```python
from build123d import *

# Parameters (mm, degrees)
F0_R     = 11
F0_R_2   = 5.5
F0_R_3   = 4
F0_R_4   = 2.9
F1_DEPTH = 1.5
F2_DEPTH = 1.65
F3_DEPTH = 5


with BuildPart() as f1:
    # F0 (on Front) → F1 (new body)
    with BuildSketch(Plane.XZ):
        Circle(F0_R)
        Circle(F0_R_2, mode=Mode.SUBTRACT)
        Circle(F0_R_2)
        Circle(F0_R_3, mode=Mode.SUBTRACT)
        Circle(F0_R_3)
        Circle(F0_R_4, mode=Mode.SUBTRACT)
        Circle(F0_R_4)
    extrude(amount=F1_DEPTH)

    # F0 (on Front) → F2 (join)
    with BuildSketch(Plane.XZ):
        Circle(F0_R_2)
        Circle(F0_R_3, mode=Mode.SUBTRACT)
    extrude(amount=F2_DEPTH)

    # F0 (on Front) → F3 (join)
    with BuildSketch(Plane.XZ):
        Circle(F0_R_3)
        Circle(F0_R_4, mode=Mode.SUBTRACT)
    extrude(amount=F3_DEPTH)


solid = f1.part
```
Input: part model. Units: mm. Frame: model coordinates. A direction names the side the tool comes from. Round coordinates to 2 decimals unless told otherwise and drop trailing zeros. Write each loop counter-clockwise with the first axis right and the second up, starting at its lowest first coordinate (ties: lowest second). Pieces come first, ordered by that corner, then holes. Notation, with made-up numbers: M -16,41 L -12,41 A9 cw -12,47 Z; hole C 22.5,-4 d2. An arc over 180 degrees is marked long. Write each question's results on one line, items separated by ' | '.
Q1. Line query: line 1 along Z through (x, y) = (0, -2.95); line 2 along Y through (x, z) = (-2.5, 6.5); line 3 along Y through (x, z) = (-4, 2.5). Output: solid intervals per line, ascending.
Results:
line 1: z = -4 to -2.9, 2.9 to 4 | line 2: y = -1.5 to 0 | line 3: y = -1.65 to 0
Q2. Draft query along X for faces 3 (the face through (-2.9, -3.2, 0.1)), 4 (the face through (0, -1.5, 0)), 5 (the face through (-4, -1.65, -2)), 6 (the face through (-2.38, -0.74, -10.74)). Return one class per face: released by +X, released by -X, zero draft, split by the parting line, or undercut.
Results:
face 3: undercut | face 4: undercut | face 5: zero draft | face 6: split by the parting line
Q3. Access query for faces 1 (the face through (-3, -1.5, 5)), 2 (the face through (0, 0, 0)). Directions: +Z, -Z, +X, -X, +Y, -Y. A direction counts if a zero-diameter tool reaches every point of the face in a straight line with its end or side. Return the directions, or none.
Results:
face 1: -Y | face 2: +Z, -Z, +X, -X, +Y
Q4. Section query B-B (x = 0). Return loops of the section in (y, z), and give its area (4 significant figures).
Results:
outline: M -5,-4 L -1.65,-4 L -1.65,-5.5 L -1.5,-5.5 L -1.5,-11 L 0,-11 L 0,11 L -1.5,11 L -1.5,5.5 L -1.65,5.5 L -1.65,4 L -5,4 L -5,2.9 L -1.5,2.9 L -1.5,-2.9 L -5,-2.9 Z | area: 41.15 mm^2
Q5. Section query D-D (y = -0.85). Return loops of the section in (x, z).
Results:
outline: C 0,0 d22
Q6. Section query A-A (z = 0). Return loops of the section in (x, y), and give its area (4 significant figures).
Results:
outline: M -11,-1.5 L -5.5,-1.5 L -5.5,-1.65 L -4,-1.65 L -4,-5 L -2.9,-5 L -2.9,-1.5 L 2.9,-1.5 L 2.9,-5 L 4,-5 L 4,-1.65 L 5.5,-1.65 L 5.5,-1.5 L 11,-1.5 L 11,0 L -11,0 Z | area: 41.15 mm^2
Q7. Section query C-C (y = -4.3). Return loops of the section in (x, z), and give its area (3 significant figures).
Results:
outline: C 0,0 d8; hole C 0,0 d5.8 | area: 23.8 mm^2
Q8. Pin query (flat end, axial travel): P1, Ø2, axis at x = -8, y = -2, coming from the -Z side; P2, Ø3.5, axis at x = 0, z = 0, coming from the -Y side. Return the tip coordinate at first contact, or that it passes through.
Results:
P1: stops at z = -8.37 | P2: stops at y = -1.5
